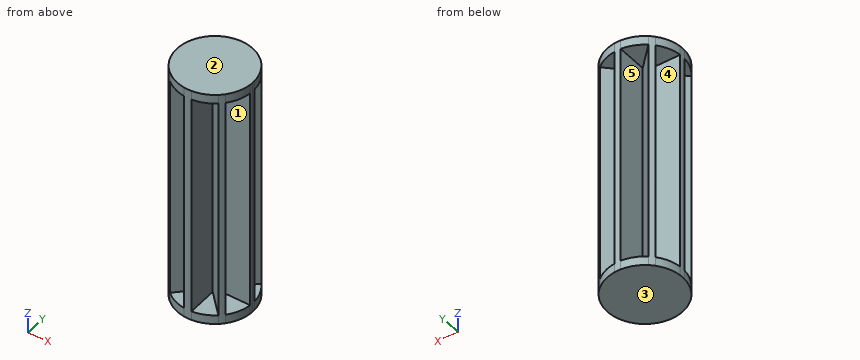
```python
from build123d import *
from build123d import SkipClean  # not in build123d's __all__

# Parameters (mm, degrees)
F1_DEPTH = 3
F2_DEPTH = 80
F4_DEPTH = 3


with BuildPart() as f1:
    # F0 (on Top) → F1 (new body)
    with BuildSketch(Plane.XY):
        with BuildLine():
            Line((1, 2.4142135624), (8.1033983122, 9.5176118745))
            ThreePointArc((8.1033983122, 9.5176118745), (4.7835429046, 11.5484941564), (1, 12.4599357944))
            Line((1, 12.4599357944), (1, 2.4142135624))
        make_face()
    extrude(amount=F1_DEPTH)



with BuildPart() as f1b:
    # F0 (on Top) → F1, piece 2 (new body)
    with BuildSketch(Plane.XY):
        with BuildLine():
            Line((-1, 2.4142135624), (-1, 12.4599357944))
            ThreePointArc((-1, 12.4599357944), (-4.7835429046, 11.5484941564), (-8.1033983122, 9.5176118745))
            Line((-8.1033983122, 9.5176118745), (-1, 2.4142135624))
        make_face()
    extrude(amount=F1_DEPTH)


with BuildPart() as f1c:
    # F0 (on Top) → F1, piece 3 (new body)
    with BuildSketch(Plane.XY):
        with BuildLine():
            Line((2.4142135624, 1), (12.4599357944, 1))
            ThreePointArc((12.4599357944, 1), (11.5484941564, 4.7835429046), (9.5176118745, 8.1033983122))
            Line((9.5176118745, 8.1033983122), (2.4142135624, 1))
        make_face()
    extrude(amount=F1_DEPTH)


with BuildPart() as f1d:
    # F0 (on Top) → F1, piece 4 (new body)
    with BuildSketch(Plane.XY):
        with BuildLine():
            ThreePointArc((9.5176118745, -8.1033983122), (11.5484941564, -4.7835429046), (12.4599357944, -1))
            Line((12.4599357944, -1), (2.4142135624, -1))
            Line((2.4142135624, -1), (9.5176118745, -8.1033983122))
        make_face()
    extrude(amount=F1_DEPTH)


with BuildPart() as f1e:
    # F0 (on Top) → F1, piece 5 (new body)
    with BuildSketch(Plane.XY):
        with BuildLine():
            Line((-12.4599357944, 1), (-2.4142135624, 1))
            Line((-2.4142135624, 1), (-9.5176118745, 8.1033983122))
            ThreePointArc((-9.5176118745, 8.1033983122), (-11.5484941564, 4.7835429046), (-12.4599357944, 1))
        make_face()
    extrude(amount=F1_DEPTH)


with BuildPart() as f1f:
    # F0 (on Top) → F1, piece 6 (new body)
    with BuildSketch(Plane.XY):
        with BuildLine():
            ThreePointArc((-12.4599357944, -1), (-11.5484941564, -4.7835429046), (-9.5176118745, -8.1033983122))
            Line((-9.5176118745, -8.1033983122), (-2.4142135624, -1))
            Line((-2.4142135624, -1), (-12.4599357944, -1))
        make_face()
    extrude(amount=F1_DEPTH)


with BuildPart() as f1g:
    # F0 (on Top) → F1, piece 7 (new body)
    with BuildSketch(Plane.XY):
        with BuildLine():
            ThreePointArc((-8.1033983122, -9.5176118745), (-4.899257332, -11.499881634), (-1.25, -12.4373429638))
            Line((-1.25, -12.4373429638), (-1, -2.4142135624))
            Line((-1, -2.4142135624), (-8.1033983122, -9.5176118745))
        make_face()
    extrude(amount=F1_DEPTH)


with BuildPart() as f1h:
    # F0 (on Top) → F1, piece 8 (new body)
    with BuildSketch(Plane.XY):
        with BuildLine():
            ThreePointArc((1.25, -12.4373429638), (4.899257332, -11.499881634), (8.1033983122, -9.5176118745))
            Line((8.1033983122, -9.5176118745), (1, -2.4142135624))
            Line((1, -2.4142135624), (1.25, -12.4373429638))
        make_face()
    extrude(amount=F1_DEPTH)


with BuildPart() as f1_1:
    add(f1.part, clean=False)

    add(f1b.part)  # F2 merges F1b

    add(f1c.part)  # F2 merges F1c

    add(f1d.part)  # F2 merges F1d

    add(f1e.part)  # F2 merges F1e

    add(f1f.part)  # F2 merges F1f

    add(f1g.part)  # F2 merges F1g

    add(f1h.part)  # F2 merges F1h
    # F0 (on Top) → F2 (join)
    with BuildSketch(Plane.XY):
        with BuildLine():
            Line((1, 2.4142135624), (1, 12.4599357944))
            ThreePointArc((1, 12.4599357944), (0, 12.5), (-1, 12.4599357944))
            Line((-1, 12.4599357944), (-1, 2.4142135624))
            Line((-1, 2.4142135624), (0, 1.4142135624))
            Line((0, 1.4142135624), (1, 2.4142135624))
        make_face()
        with BuildLine():
            Line((2.4142135624, 1), (9.5176118745, 8.1033983122))
            ThreePointArc((9.5176118745, 8.1033983122), (8.8388347648, 8.8388347648), (8.1033983122, 9.5176118745))
            Line((8.1033983122, 9.5176118745), (1, 2.4142135624))
            Line((1, 2.4142135624), (0, 1.4142135624))
            Line((0, 1.4142135624), (-1, 2.4142135624))
            Line((-1, 2.4142135624), (-8.1033983122, 9.5176118745))
            ThreePointArc((-8.1033983122, 9.5176118745), (-8.8388347648, 8.8388347648), (-9.5176118745, 8.1033983122))
            Line((-9.5176118745, 8.1033983122), (-2.4142135624, 1))
            Line((-2.4142135624, 1), (0, -1.4142135624))
            Line((0, -1.4142135624), (1, -2.4142135624))
            Line((1, -2.4142135624), (8.1033983122, -9.5176118745))
            ThreePointArc((8.1033983122, -9.5176118745), (8.8388347648, -8.8388347648), (9.5176118745, -8.1033983122))
            Line((9.5176118745, -8.1033983122), (2.4142135624, -1))
            Line((2.4142135624, -1), (1.4142135624, 0))
            Line((1.4142135624, 0), (2.4142135624, 1))
        make_face()
        with BuildLine():
            Line((-1, -2.4142135624), (0, -1.4142135624))
            Line((0, -1.4142135624), (-2.4142135624, 1))
            Line((-2.4142135624, 1), (-12.4599357944, 1))
            ThreePointArc((-12.4599357944, 1), (-12.5, 0), (-12.4599357944, -1))
            Line((-12.4599357944, -1), (-2.4142135624, -1))
            Line((-2.4142135624, -1), (-9.5176118745, -8.1033983122))
            ThreePointArc((-9.5176118745, -8.1033983122), (-8.8388347648, -8.8388347648), (-8.1033983122, -9.5176118745))
            Line((-8.1033983122, -9.5176118745), (-1, -2.4142135624))
        make_face()
        with BuildLine():
            ThreePointArc((12.4599357944, -1), (12.4899799325, -0.5004011242), (12.5, 0))
            ThreePointArc((12.5, 0), (12.4899799325, 0.5004011242), (12.4599357944, 1))
            Line((12.4599357944, 1), (2.4142135624, 1))
            Line((2.4142135624, 1), (1.4142135624, 0))
            Line((1.4142135624, 0), (2.4142135624, -1))
            Line((2.4142135624, -1), (12.4599357944, -1))
        make_face()
        with BuildLine():
            ThreePointArc((-1.25, -12.4373429638), (0, -12.5), (1.25, -12.4373429638))
            Line((1.25, -12.4373429638), (1, -2.4142135624))
            Line((1, -2.4142135624), (0, -1.4142135624))
            Line((0, -1.4142135624), (-1, -2.4142135624))
            Line((-1, -2.4142135624), (-1.25, -12.4373429638))
        make_face()
    extrude(amount=F2_DEPTH)

    # F3 (on face) → F4 (join)
    with BuildSketch(Plane.XY.offset(80)):
        with BuildLine():
            Line((1, 2.4142135624), (8.1033983122, 9.5176118745))
            ThreePointArc((8.1033983122, 9.5176118745), (4.7835429046, 11.5484941564), (1, 12.4599357944))
            Line((1, 12.4599357944), (1, 2.4142135624))
        make_face()
        with BuildLine():
            Line((-1, 2.4142135624), (-1, 12.4599357944))
            ThreePointArc((-1, 12.4599357944), (-4.7835429046, 11.5484941564), (-8.1033983122, 9.5176118745))
            Line((-8.1033983122, 9.5176118745), (-1, 2.4142135624))
        make_face()
        with BuildLine():
            ThreePointArc((12.4599357944, -1), (12.4899799325, -0.5004011242), (12.5, 0))
            ThreePointArc((12.5, 0), (12.4899799325, 0.5004011242), (12.4599357944, 1))
            Line((12.4599357944, 1), (2.4142135624, 1))
            Line((2.4142135624, 1), (9.5176118745, 8.1033983122))
            ThreePointArc((9.5176118745, 8.1033983122), (8.8388347648, 8.8388347648), (8.1033983122, 9.5176118745))
            Line((8.1033983122, 9.5176118745), (1, 2.4142135624))
            Line((1, 2.4142135624), (1, 12.4599357944))
            ThreePointArc((1, 12.4599357944), (0, 12.5), (-1, 12.4599357944))
            Line((-1, 12.4599357944), (-1, 2.4142135624))
            Line((-1, 2.4142135624), (-8.1033983122, 9.5176118745))
            ThreePointArc((-8.1033983122, 9.5176118745), (-8.8388347648, 8.8388347648), (-9.5176118745, 8.1033983122))
            Line((-9.5176118745, 8.1033983122), (-2.4142135624, 1))
            Line((-2.4142135624, 1), (-12.4599357944, 1))
            ThreePointArc((-12.4599357944, 1), (-12.5, 0), (-12.4599357944, -1))
            Line((-12.4599357944, -1), (-2.4142135624, -1))
            Line((-2.4142135624, -1), (-9.5176118745, -8.1033983122))
            ThreePointArc((-9.5176118745, -8.1033983122), (-8.8388347648, -8.8388347648), (-8.1033983122, -9.5176118745))
            Line((-8.1033983122, -9.5176118745), (-1, -2.4142135624))
            Line((-1, -2.4142135624), (-1.25, -12.4373429638))
            ThreePointArc((-1.25, -12.4373429638), (0, -12.5), (1.25, -12.4373429638))
            Line((1.25, -12.4373429638), (1, -2.4142135624))
            Line((1, -2.4142135624), (8.1033983122, -9.5176118745))
            ThreePointArc((8.1033983122, -9.5176118745), (8.8388347648, -8.8388347648), (9.5176118745, -8.1033983122))
            Line((9.5176118745, -8.1033983122), (2.4142135624, -1))
            Line((2.4142135624, -1), (12.4599357944, -1))
        make_face()
        with BuildLine():
            Line((-2.4142135624, 1), (-9.5176118745, 8.1033983122))
            ThreePointArc((-9.5176118745, 8.1033983122), (-11.5484941564, 4.7835429046), (-12.4599357944, 1))
            Line((-12.4599357944, 1), (-2.4142135624, 1))
        make_face()
        with BuildLine():
            ThreePointArc((-12.4599357944, -1), (-11.5484941564, -4.7835429046), (-9.5176118745, -8.1033983122))
            Line((-9.5176118745, -8.1033983122), (-2.4142135624, -1))
            Line((-2.4142135624, -1), (-12.4599357944, -1))
        make_face()
        with BuildLine():
            ThreePointArc((-8.1033983122, -9.5176118745), (-4.899257332, -11.499881634), (-1.25, -12.4373429638))
            Line((-1.25, -12.4373429638), (-1, -2.4142135624))
            Line((-1, -2.4142135624), (-8.1033983122, -9.5176118745))
        make_face()
        with BuildLine():
            ThreePointArc((1.25, -12.4373429638), (4.899257332, -11.499881634), (8.1033983122, -9.5176118745))
            Line((8.1033983122, -9.5176118745), (1, -2.4142135624))
            Line((1, -2.4142135624), (1.25, -12.4373429638))
        make_face()
        with BuildLine():
            ThreePointArc((9.5176118745, -8.1033983122), (11.5484941564, -4.7835429046), (12.4599357944, -1))
            Line((12.4599357944, -1), (2.4142135624, -1))
            Line((2.4142135624, -1), (9.5176118745, -8.1033983122))
        make_face()
        with BuildLine():
            Line((2.4142135624, 1), (12.4599357944, 1))
            ThreePointArc((12.4599357944, 1), (11.5484941564, 4.7835429046), (9.5176118745, 8.1033983122))
            Line((9.5176118745, 8.1033983122), (2.4142135624, 1))
        make_face()
    with SkipClean():  # cleaning this boolean's faces spoils the solid; the shape is the same uncleaned
        extrude(amount=-F4_DEPTH)


solid = f1_1.part
```
Geometry: final body of the model. Coordinates: model frame, mm. Face numbers are marked on the shaded views. A direction names the side the tool comes from. Give positions to 0.01 mm unless a question says otherwise; leave off trailing zeros. Loops run counter-clockwise (first coordinate to the right, second up) from the corner with the lowest first, then second, coordinate; pieces in that order, holes last. Notation, with made-up numbers: (36, -22.5) - (94, -22.5) arc R16 cw to (94, -17.5) - close; hole circle Ø2 at (29.25, -6). An arc over 180 degrees is marked (long way). Answer as CSV lines item,"result". Start each with the question number.
(1) Pin query (flat end, axial travel): P1, Ø4, axis at x = -6, z = 42, coming from the -Y side; P2, Ø3, axis at y = 9, z = 30.5, coming from the -X side; P3, Ø6, axis at x = -6, z = 32.5, coming from the -Y side. Return the tip coordinate at first contact, or that it passes through.
(2) Reachability of the marked faces 4 and 5 from +Z, -Z, +X, -X, +Y, -Y: full face, straight path, thin tool, end or side. Return the list, or none.
(3) Ray query, line 1 along Z through (x, y) = (8.25, 5.5); line 2 along X through (y, z) = (-6, 61); line 3 along Y through (x, z) = (5.25, 29). Return the intervals inside material, ascending. Write a range as [from, to].
(4) Mould query, pull axis Z, two halves, no side actions, for the marked faces 1, 2 and 3. Classes: +Z half, -Z half, draft (parallel to the pull), parting line (faces both ways), or undercut.
(5) Section query B-B (y = -6.5). Output: boundary loops of the cut face in (x, z), and give its area (3 significant figures).
(6) Section query C-C (z = 70). Output: boundary loops of the cut face in (x, y), and give its area (3 significant figures).
(7) Section query A-A (x = 6.5). Output: boundary loops of the cut face in (y, z), and give its area (3 significant figures).
Worked answers:
1,P1,"stops at y = -9.41"
1,P2,"stops at x = -9.52"
1,P3,"stops at y = -9.52"
2,face 4,"-X"
2,face 5,"+Y"
3,line 1,"z = [0, 3], [77, 80]"
3,line 2,"x = [-7.41, -4.59], [-1.09, 1.09], [4.59, 7.41]"
3,line 3,"y = [-6.66, -3.84], [-1, 1], [3.84, 6.66]"
4,face 1,"undercut"
4,face 2,"+Z half"
4,face 3,"-Z half"
5,outline,"(-10.68, 0) - (10.68, 0) - (10.68, 3) - (7.91, 3) - (7.91, 77) - (10.68, 77) - (10.68, 80) - (-10.68, 80) - (-10.68, 77) - (-7.91, 77) - (-7.91, 3) - (-10.68, 3) - close; hole (-5.09, 3) - (-1.1, 3) - (-1.1, 77) - (-5.09, 77) - close; hole (1.1, 3) - (5.09, 3) - (5.09, 77) - (1.1, 77) - close"
5,area,"710 mm^2"
6,outline,"(-12.46, -1) - (-2.41, -1) - (-9.52, -8.1) arc R12.5 ccw to (-8.1, -9.52) - (-1, -2.41) - (-1.25, -12.44) arc R12.5 ccw to (1.25, -12.44) - (1, -2.41) - (8.1, -9.52) arc R12.5 ccw to (9.52, -8.1) - (2.41, -1) - (12.46, -1) arc R12.5 ccw to (12.46, 1) - (2.41, 1) - (9.52, 8.1) arc R12.5 ccw to (8.1, 9.52) - (1, 2.41) - (1, 12.46) arc R12.5 ccw to (-1, 12.46) - (-1, 2.41) - (-8.1, 9.52) arc R12.5 ccw to (-9.52, 8.1) - (-2.41, 1) - (-12.46, 1) arc R12.5 ccw to start"
6,area,"183 mm^2"
7,outline,"(-10.68, 0) - (10.68, 0) - (10.68, 3) - (7.91, 3) - (7.91, 77) - (10.68, 77) - (10.68, 80) - (-10.68, 80) - (-10.68, 77) - (-7.91, 77) - (-7.91, 3) - (-10.68, 3) - close; hole (-5.09, 3) - (-1, 3) - (-1, 77) - (-5.09, 77) - close; hole (1, 3) - (5.09, 3) - (5.09, 77) - (1, 77) - close"
7,area,"695 mm^2"
